For this review, take the finished solid that the model builds, in its own axes (mm). A direction names the side the tool comes from. Coordinates: 2 decimals unless noted, no trailing zeros. Loops run counter-clockwise (first coordinate to the right, second up) from the corner with the lowest first, then second, coordinate; pieces in that order, holes last. Notation, with made-up numbers: M 13,66 L 66,66 A29 ccw 66,90 Z; hole C 78,17.5 d8. An arc over 180 degrees is marked long. Write item = value, one per line.
from build123d import *

# Parameters (mm, degrees)
BOSS_EXTRU_1_DEPTH         = 100
PER_AGEAVANC_1_START       = -1
PER_AGEAVANC_1_OUTLINE_R   = 3
PER_AGEAVANC_1_DEPTH       = 5
PER_AGEAVANC_1_START_2     = -4
PER_AGEAVANC_1_2_OUTLINE_R = 1.7
PER_AGEAVANC_1_2_DEPTH     = 3


# Read off the part's stored shape, not the designer's step: PerçageAvancé1
with BuildPart() as part:
    # Esquisse1 → Boss.-Extru.1 (new, symmetric)
    with BuildSketch(Plane.XY):
        Polygon((6, 2), (6, 4), (-6, 4), (-6, 2), (-4, 2), (-4, 1), (-6, 1), (-6, -4), (6, -4), (6, 1), (4, 1), (4, 2), align=None)
    extrude(amount=BOSS_EXTRU_1_DEPTH, both=True)

    # PerçageAvancé1 outline → PerçageAvancé1 (cut)
    with BuildSketch(Plane(origin=(0, 0, 0), x_dir=(1, 0, 0), z_dir=(0, 1, 0)).offset(PER_AGEAVANC_1_START)):
        with Locations((0, -87.5)):
            Circle(PER_AGEAVANC_1_OUTLINE_R)
        with Locations((0, -62.5)):
            Circle(PER_AGEAVANC_1_OUTLINE_R)
        with Locations((0, -37.5)):
            Circle(PER_AGEAVANC_1_OUTLINE_R)
        with Locations((0, -12.5)):
            Circle(PER_AGEAVANC_1_OUTLINE_R)
        with Locations((0, 12.5)):
            Circle(PER_AGEAVANC_1_OUTLINE_R)
        with Locations((0, 87.5)):
            Circle(PER_AGEAVANC_1_OUTLINE_R)
        with Locations((0, 62.5)):
            Circle(PER_AGEAVANC_1_OUTLINE_R)
        with Locations((0, 37.5)):
            Circle(PER_AGEAVANC_1_OUTLINE_R)
    extrude(amount=PER_AGEAVANC_1_DEPTH, mode=Mode.SUBTRACT)

    # Per_ageAvanc_1 2 outline → Per_ageAvanc_1 2 (cut)
    with BuildSketch(Plane(origin=(0, 0, 0), x_dir=(1, 0, 0), z_dir=(0, 1, 0)).offset(PER_AGEAVANC_1_START_2)):
        with Locations((0, -87.5)):
            Circle(PER_AGEAVANC_1_2_OUTLINE_R)
        with Locations((0, -62.5)):
            Circle(PER_AGEAVANC_1_2_OUTLINE_R)
        with Locations((0, -37.5)):
            Circle(PER_AGEAVANC_1_2_OUTLINE_R)
        with Locations((0, -12.5)):
            Circle(PER_AGEAVANC_1_2_OUTLINE_R)
        with Locations((0, 12.5)):
            Circle(PER_AGEAVANC_1_2_OUTLINE_R)
        with Locations((0, 87.5)):
            Circle(PER_AGEAVANC_1_2_OUTLINE_R)
        with Locations((0, 62.5)):
            Circle(PER_AGEAVANC_1_2_OUTLINE_R)
        with Locations((0, 37.5)):
            Circle(PER_AGEAVANC_1_2_OUTLINE_R)
    extrude(amount=PER_AGEAVANC_1_2_DEPTH, mode=Mode.SUBTRACT)


solid = part.part
Q1. Draft analysis for pull direction X (two halves, no side actions). For faces 3 (the face through (-0.391, 1.465, 34.526)), 4 (the face through (0, -4, 1)), 5 (the face through (-6, -1, 1)), state which applies: +X half, -X half, draft (parallel to the pull), parting line (faces both ways), or undercut.
Solved:
face_3 = undercut
face_4 = draft
face_5 = -X half
Q2. Machinability: for faces 1 (the face through (2, -1, 87)), 2 (the face through (-0.221, -2.521, 60.814)), which of the approach directions +Z, -Z, +X, -X, +Y, -Y give a long, thin tool a straight path to every point of the face, cutting with its end or side? Answer none if there is none.
Solved:
face_1 = +Y
face_2 = +Y, -Y
Q3. Add section A-A (z = -12.5). Write out the cut boundary in (x, y), and give its area (3 significant figures).
Solved:
outline = M -6,-4 L -1.7,-4 L -1.7,-1 L -3,-1 L -3,4 L -6,4 L -6,2 L -4,2 L -4,1 L -6,1 Z; M 1.7,-4 L 6,-4 L 6,1 L 4,1 L 4,2 L 6,2 L 6,4 L 3,4 L 3,-1 L 1.7,-1 Z
area = 51.8 mm²
Q4. Add section B-B (y = -2.75). State how many separate pieces and enclosed holes the cut face has, and give its area (3 significant figures).
Solved:
separate_pieces = 1
enclosed_holes = 8
area = 2,330 mm²
Q5. For line 1 along Y through (x, z) = (-5.5, -83); line 2 along X through (y, z) = (0.5, -37.5); line 3 along X through (y, z) = (-3, 12.5), list the stretches that pass through material, from the lowest coordinate up.
Solved:
line_1 = -4 to 1, 2 to 4
line_2 = -6 to -3, 3 to 6
line_3 = -6 to -1.7, 1.7 to 6
Q6. For pin 1 Ø1.8 at (x, z) = (-0.5, 87) entering from +Y; pin 2 Ø3 at (x, z) = (1, -62) entering from +Y, all flat-tipped, find the tip position at first contact; note any pin that passes through.
Solved:
pin_1 = through
pin_2 = -1
